```python
from build123d import *

# Parameters (mm, degrees)
BOSS_EXTRUDE1_DEPTH = 3
CUT_EXTRUDE1_DEPTH  = 0.5
SKETCH3_W           = 5
SKETCH3_H           = 0.5
SKETCH4_W           = 5
SKETCH4_H           = 0.5
SKETCH5_W           = 5
SKETCH5_H           = 0.5
CUT_EXTRUDE2_DEPTH  = 0.5
CUT_EXTRUDE3_DEPTH  = 0.5
CUT_EXTRUDE4_DEPTH  = 0.5
CUT_EXTRUDE5_DEPTH  = 0.5
BOSS_EXTRUDE2_DEPTH = 8
BOSS_EXTRUDE3_DEPTH = 8
BOSS_EXTRUDE4_DEPTH = 8
SKETCH16_W          = 0.75
SKETCH16_H          = 8
SKETCH17_W          = 0.75
SKETCH17_H          = 8
SKETCH18_W          = 0.75
SKETCH18_H          = 8


with BuildPart() as part:
    # Sketch1 → Boss-Extrude1 (new body)
    with BuildSketch(Plane.XY):
        with BuildLine():
            Line((-29, -10), (29, -10))
            ThreePointArc((29, -10), (29.707106781, -9.707106781), (30, -9))
            Line((30, -9), (30, 9))
            ThreePointArc((30, 9), (29.707106781, 9.707106781), (29, 10))
            Line((29, 10), (-29, 10))
            ThreePointArc((-29, 10), (-29.707106781, 9.707106781), (-30, 9))
            Line((-30, 9), (-30, -9))
            ThreePointArc((-30, -9), (-29.707106781, -9.707106781), (-29, -10))
        make_face()
    extrude(amount=-BOSS_EXTRUDE1_DEPTH)

    # Sketch2 → Cut-Extrude1 (cut)
    with BuildSketch(Plane.XY):
        with BuildLine():
            Line((-25.75, -8.75), (25.75, -8.75))
            ThreePointArc((25.75, -8.75), (27.871320344, -7.871320344), (28.75, -5.75))
            Line((28.75, -5.75), (28.75, 5.75))
            ThreePointArc((28.75, 5.75), (27.871320344, 7.871320344), (25.75, 8.75))
            Line((25.75, 8.75), (-25.75, 8.75))
            ThreePointArc((-25.75, 8.75), (-27.871320344, 7.871320344), (-28.75, 5.75))
            Line((-28.75, 5.75), (-28.75, -5.75))
            ThreePointArc((-28.75, -5.75), (-27.871320344, -7.871320344), (-25.75, -8.75))
        make_face()
    extrude(amount=-CUT_EXTRUDE1_DEPTH, mode=Mode.SUBTRACT)

    # Sketch3 → Cut-Revolve1 (revolve, cut)
    with BuildSketch(Plane(origin=(0, 0, 0), x_dir=(1, 0, 0), z_dir=(0, 1, 0)), mode=Mode.PRIVATE) as cut_revolve1_sk:
        with Locations((-17.75, 0.75)):
            Rectangle(SKETCH3_W, SKETCH3_H)
    revolve(cut_revolve1_sk.sketch.rotate(Axis((-20.25, 0, -0.5), (0, 0, -1)), 180), axis=Axis((-20.25, 0, -0.5), (0, 0, -1)), mode=Mode.SUBTRACT)

    # Sketch4 → Cut-Revolve2 (revolve, cut)
    with BuildSketch(Plane(origin=(0, 0, 0), x_dir=(1, 0, 0), z_dir=(0, 1, 0)), mode=Mode.PRIVATE) as cut_revolve2_sk:
        with Locations((2.5, 0.75)):
            Rectangle(SKETCH4_W, SKETCH4_H)
    revolve(cut_revolve2_sk.sketch.rotate(Axis((0, 0, -0.5), (0, 0, -1)), 180), axis=Axis((0, 0, -0.5), (0, 0, -1)), mode=Mode.SUBTRACT)

    # Sketch5 → Cut-Revolve3 (revolve, cut)
    with BuildSketch(Plane(origin=(0, 0, 0), x_dir=(1, 0, 0), z_dir=(0, 1, 0)), mode=Mode.PRIVATE) as cut_revolve3_sk:
        with Locations((22.75, 0.75)):
            Rectangle(SKETCH5_W, SKETCH5_H)
    revolve(cut_revolve3_sk.sketch.rotate(Axis((20.25, 0, -0.5), (0, 0, -1)), 180), axis=Axis((20.25, 0, -0.5), (0, 0, -1)), mode=Mode.SUBTRACT)

    # Sketch6 → Cut-Extrude2 (cut)
    with BuildSketch(Plane.XY.offset(-0.5)):
        with BuildLine():
            Line((-9.031754163, 8.75), (-10.968245837, 8.75))
            ThreePointArc((-10.968245837, 8.75), (-10, 5), (-9.031754163, 8.75))
        make_face()
    extrude(amount=-CUT_EXTRUDE2_DEPTH, mode=Mode.SUBTRACT)

    # Sketch7 → Cut-Extrude3 (cut)
    with BuildSketch(Plane.XY.offset(-0.5)):
        with BuildLine():
            Line((10.968245837, 8.75), (9.031754163, 8.75))
            ThreePointArc((9.031754163, 8.75), (10, 5), (10.968245837, 8.75))
        make_face()
    extrude(amount=-CUT_EXTRUDE3_DEPTH, mode=Mode.SUBTRACT)

    # Sketch8 → Cut-Extrude4 (cut)
    with BuildSketch(Plane.XY.offset(-0.5)):
        with BuildLine():
            Line((-10.968245837, -8.75), (-9.031754163, -8.75))
            ThreePointArc((-9.031754163, -8.75), (-10, -5), (-10.968245837, -8.75))
        make_face()
    extrude(amount=-CUT_EXTRUDE4_DEPTH, mode=Mode.SUBTRACT)

    # Sketch9 → Cut-Extrude5 (cut)
    with BuildSketch(Plane.XY.offset(-0.5)):
        with BuildLine():
            Line((9.031754163, -8.75), (10.968245837, -8.75))
            ThreePointArc((10.968245837, -8.75), (10, -5), (9.031754163, -8.75))
        make_face()
    extrude(amount=-CUT_EXTRUDE5_DEPTH, mode=Mode.SUBTRACT)

    # Sketch10 → Boss-Extrude2 (add)
    with BuildSketch(Plane.XY.offset(-1)):
        with BuildLine():
            Line((-1.13937326, -1.193452376), (-1.409978177, -1.94215384))
            ThreePointArc((-1.409978177, -1.94215384), (-1.2, -2.078460969), (-0.976965475, -2.19215384))
            Line((-0.976965475, -2.19215384), (-0.463873445, -1.583452376))
            ThreePointArc((-0.463873445, -1.583452376), (0.825, -1.428941916), (1.603246706, -0.39))
            Line((1.603246706, -0.39), (2.386943652, -0.25))
            ThreePointArc((2.386943652, -0.25), (2.4, 0), (2.386943652, 0.25))
            Line((2.386943652, 0.25), (1.603246706, 0.39))
            ThreePointArc((1.603246706, 0.39), (0.825, 1.428941916), (-0.463873445, 1.583452376))
            Line((-0.463873445, 1.583452376), (-0.976965475, 2.19215384))
            ThreePointArc((-0.976965475, 2.19215384), (-1.2, 2.078460969), (-1.409978177, 1.94215384))
            Line((-1.409978177, 1.94215384), (-1.13937326, 1.193452376))
            ThreePointArc((-1.13937326, 1.193452376), (-1.65, 0), (-1.13937326, -1.193452376))
        make_face()
    extrude(amount=BOSS_EXTRUDE2_DEPTH)

    # Sketch11 → Boss-Extrude3 (add)
    with BuildSketch(Plane.XY.offset(-1)):
        with BuildLine():
            Line((-21.38937326, -1.193452376), (-21.659978177, -1.94215384))
            ThreePointArc((-21.659978177, -1.94215384), (-21.45, -2.078460969), (-21.226965475, -2.19215384))
            Line((-21.226965475, -2.19215384), (-20.713873445, -1.583452376))
            ThreePointArc((-20.713873445, -1.583452376), (-19.425, -1.428941916), (-18.646753294, -0.39))
            Line((-18.646753294, -0.39), (-17.863056348, -0.25))
            ThreePointArc((-17.863056348, -0.25), (-17.85, 0), (-17.863056348, 0.25))
            Line((-17.863056348, 0.25), (-18.646753294, 0.39))
            ThreePointArc((-18.646753294, 0.39), (-19.425, 1.428941916), (-20.713873445, 1.583452376))
            Line((-20.713873445, 1.583452376), (-21.226965475, 2.19215384))
            ThreePointArc((-21.226965475, 2.19215384), (-21.45, 2.078460969), (-21.659978177, 1.94215384))
            Line((-21.659978177, 1.94215384), (-21.38937326, 1.193452376))
            ThreePointArc((-21.38937326, 1.193452376), (-21.9, 0), (-21.38937326, -1.193452376))
        make_face()
    extrude(amount=BOSS_EXTRUDE3_DEPTH)

    # Sketch12 → Boss-Extrude4 (add)
    with BuildSketch(Plane.XY.offset(-1)):
        with BuildLine():
            Line((17.863056348, -0.25), (18.646753294, -0.39))
            ThreePointArc((18.646753294, -0.39), (19.425, -1.428941916), (20.713873445, -1.583452376))
            Line((20.713873445, -1.583452376), (21.226965475, -2.19215384))
            ThreePointArc((21.226965475, -2.19215384), (21.45, -2.078460969), (21.659978177, -1.94215384))
            Line((21.659978177, -1.94215384), (21.38937326, -1.193452376))
            ThreePointArc((21.38937326, -1.193452376), (21.9, 0), (21.38937326, 1.193452376))
            Line((21.38937326, 1.193452376), (21.659978177, 1.94215384))
            ThreePointArc((21.659978177, 1.94215384), (21.45, 2.078460969), (21.226965475, 2.19215384))
            Line((21.226965475, 2.19215384), (20.713873445, 1.583452376))
            ThreePointArc((20.713873445, 1.583452376), (19.425, 1.428941916), (18.646753294, 0.39))
            Line((18.646753294, 0.39), (17.863056348, 0.25))
            ThreePointArc((17.863056348, 0.25), (17.85, 0), (17.863056348, -0.25))
        make_face()
    extrude(amount=BOSS_EXTRUDE4_DEPTH)

    # Sketch13 → Cut-Revolve4 (revolve, cut)
    with BuildSketch(Plane(origin=(0, 0, 0), x_dir=(1, 0, 0), z_dir=(0, 1, 0))):
        Polygon((-18.7125, -7.3), (-17.55, -7.3), (-17.55, -4.2), align=None)
    revolve(axis=Axis((-20.25, 0, 50), (0, 0, -1)), mode=Mode.SUBTRACT)

    # Sketch14 → Cut-Revolve5 (revolve, cut)
    with BuildSketch(Plane(origin=(0, 0, 0), x_dir=(1, 0, 0), z_dir=(0, 1, 0))):
        Polygon((1.5375, -7.3), (2.7, -7.3), (2.7, -4.2), align=None)
    revolve(axis=Axis((0, 0, 50), (0, 0, -1)), mode=Mode.SUBTRACT)

    # Sketch15 → Cut-Revolve6 (revolve, cut)
    with BuildSketch(Plane(origin=(0, 0, 0), x_dir=(1, 0, 0), z_dir=(0, 1, 0))):
        Polygon((21.7875, -7.3), (22.95, -7.3), (22.95, -4.2), align=None)
    revolve(axis=Axis((20.25, 0, 50), (0, 0, -1)), mode=Mode.SUBTRACT)

    # Sketch16 → Cut-Revolve7 (revolve, cut)
    with BuildSketch(Plane(origin=(0, 0, 0), x_dir=(1, 0, 0), z_dir=(0, 1, 0)), mode=Mode.PRIVATE) as cut_revolve7_sk:
        with Locations((-19.875, -3)):
            Rectangle(SKETCH16_W, SKETCH16_H)
    revolve(cut_revolve7_sk.sketch.rotate(Axis((-20.25, 0, 7), (0, 0, -1)), 180), axis=Axis((-20.25, 0, 7), (0, 0, -1)), mode=Mode.SUBTRACT)

    # Sketch17 → Cut-Revolve8 (revolve, cut)
    with BuildSketch(Plane(origin=(0, 0, 0), x_dir=(1, 0, 0), z_dir=(0, 1, 0)), mode=Mode.PRIVATE) as cut_revolve8_sk:
        with Locations((0.375, -3)):
            Rectangle(SKETCH17_W, SKETCH17_H)
    revolve(cut_revolve8_sk.sketch.rotate(Axis((0, 0, 7), (0, 0, -1)), 180), axis=Axis((0, 0, 7), (0, 0, -1)), mode=Mode.SUBTRACT)

    # Sketch18 → Cut-Revolve9 (revolve, cut)
    with BuildSketch(Plane(origin=(0, 0, 0), x_dir=(1, 0, 0), z_dir=(0, 1, 0)), mode=Mode.PRIVATE) as cut_revolve9_sk:
        with Locations((20.625, -3)):
            Rectangle(SKETCH18_W, SKETCH18_H)
    revolve(cut_revolve9_sk.sketch.rotate(Axis((20.25, 0, 7), (0, 0, -1)), 180), axis=Axis((20.25, 0, 7), (0, 0, -1)), mode=Mode.SUBTRACT)


solid = part.part
```
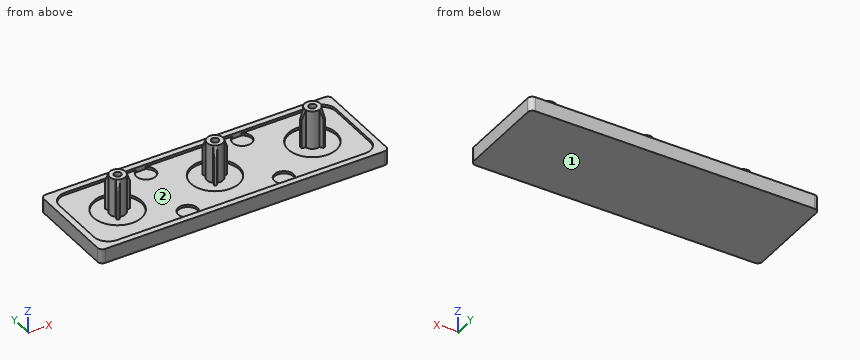
Design review of the part built by this model. Coordinates are the model's own, in mm. Face numbers are marked on the shaded views. Give positions to 0.01 mm unless a question says otherwise; leave off trailing zeros. Write each loop counter-clockwise with the first axis right and the second up, starting at its lowest first coordinate (ties: lowest second). Pieces come first, ordered by that corner, then holes. Notation, with made-up numbers: (-37, 51) - (-11, 51) arc R14 cw to (-11, 75) - close; hole circle Ø11 at (85.25, 87.25). An arc over 180 degrees is marked (long way). Return JSON: item names as keys, results as strings. Group by question number.
(1) We need section A-A, the plane y = -3. Give the boundary of the cut face in (x, z).
(2) We need section B-B, the plane x = 7. Give the boundary of the cut face in (y, z), then the cut area to 4 significant figures.
(3) Insertion check: pin 1 (5 mm diameter, centred on x = 5, y = 4.5, fed in from +Z); pin 2 (1.1 mm diameter, centred on x = 10.5, y = -6.5, fed in from +Z); pin 3 (8 mm diameter, centred on x = 22.5, y = 0.5, fed in from +Z); pin 4 (4 mm diameter, centred on x = -10, y = 7.5, fed in from +Z). Each pin has a flat end and moves straight along its axis. Give the tip position at first contact, or say it passes through.
(4) We need section D-D, the plane x = -10. Give the boundary of the cut face in (y, z).
(5) Mouldability with a two-part tool opening along Y and no side actions: class the marked faces 1 and 2 as +Y half, -Y half, draft (parallel to the pull), parting line (faces both ways), or undercut.
(6) To check wall thickness, follow probe 1 along Y at (x, z) = (20.25, -0.55); probe 2 along Y at (x, z) = (10, -0.7); probe 3 along X at (y, z) = (-7, -0.7). State the ranges of each line that lie inside material, in increasing order.
(7) We need section C-C, the plane z = 1.5. Give the number of separate pieces and of enclosed holes in the cut face, then the cut area to 3 significant figures.
Reported:
{
 "1": {"outline": "(-30, -3) - (30, -3) - (30, 0) - (28.75, 0) - (28.75, -0.5) - (24.25, -0.5) - (24.25, -1) - (16.25, -1) - (16.25, -0.5) - (4, -0.5) - (4, -1) - (-4, -1) - (-4, -0.5) - (-16.25, -0.5) - (-16.25, -1) - (-24.25, -1) - (-24.25, -0.5) - (-28.75, -0.5) - (-28.75, 0) - (-30, 0) - close"},
 "2": {"outline": "(-10, -3) - (10, -3) - (10, 0) - (8.75, 0) - (8.75, -0.5) - (-8.75, -0.5) - (-8.75, 0) - (-10, 0) - close", "area": "51.25 mm2"},
 "3": {"pin 1": "stops at z = -0.5", "pin 2": "stops at z = -1", "pin 3": "stops at z = 7", "pin 4": "stops at z = 0"},
 "4": {"outline": "(-10, -3) - (10, -3) - (10, 0) - (8.75, 0) - (8.75, -1) - (5, -1) - (5, -0.5) - (-5, -0.5) - (-5, -1) - (-8.75, -1) - (-8.75, 0) - (-10, 0) - close"},
 "5": {"face 1": "draft", "face 2": "undercut"},
 "6": {"probe 1": "y = -10 to -5, -1.65 to -0.75, 0.75 to 1.65, 5 to 10", "probe 2": "y = -10 to -8.75, -5 to 5, 8.75 to 10", "probe 3": "x = -30 to -12, -8 to 8, 12 to 30"},
 "7": {"separate pieces": "3", "enclosed holes": "3", "area": "24.7 mm2"}
}
